Input: part model. Units: mm. Frame: model coordinates. A direction names the side the tool comes from. Coordinates: 2 decimals unless noted, no trailing zeros. Loops run counter-clockwise (first coordinate to the right, second up) from the corner with the lowest first, then second, coordinate; pieces in that order, holes last. Notation, with made-up numbers: (-6, -27.5) - (1, -27.5) arc R30 cw to (1, 10.5) - close; hole circle Ø11 at (-7.5, -29.5). An arc over 180 degrees is marked (long way). Use a Markdown table: item, result. Add a question column.
1. Section query C-C on z = -18. Return the cut outline in (x, y) (3 decimals), then the cut area to 3 significant figures.
2. Contact query for flat-ended pins moving along their axis: P1, Ø4, axis at x = 34.5, y = 0, coming from the -Z side (3 decimals); P2, Ø1.5, axis at y = 2, z = -17.5, coming from the +X side (3 decimals); P3, Ø4, axis at y = -2.5, z = -18.5, coming from the -X side (3 decimals). Output: stop coordinate, or through.
3. Access query for faces 4 (the face through (26, 0, -15.875)), 5 (the face through (45, 0, 15.875)), 6 (the face through (-27, 0, -15.875)). Directions: +Z, -Z, +X, -X, +Y, -Y. A direction counts if a zero-diameter tool reaches every point of the face in a straight line with its end or side. Return the directions, or none.
4. Section query A-A on z = 13.5. Return the cut outline in (x, y), then the cut area to 3 significant figures.
5. Section query B-B on y = 1.75. Return the cut outline in (x, z) (3 decimals), then the cut area to 3 significant figures.
6. Ray query, L1, parallel to X at y = -4, z = -16.5 (3 decimals); L2, parallel to Z at x = -42, y = -2 (3 decimals); L3, parallel to X at y = -2.75, z = 6.5. Return the intervals inside material, ascending. Write a range as [from, to].
7. Draft query along X for faces 1 (the face through (-0.63, -0.09, -3.17)), 2 (the face through (50.8, 0, 0)), 3 (the face through (-45, 0, 15.875)). Return one class per face: released by +X, released by -X, zero draft, split by the parting line, or undercut.
8. Section query D-D on x = 43.5. Return the cut outline in (y, z) (3 decimals), then the cut area to 3 significant figures.
```python
from build123d import *

# Parameters (mm, degrees)
F0_W     = 101.6
F0_H     = 31.75
F1_DEPTH = 6.35
F3_DEPTH = 12.7
F4_W     = 6.35
F4_H     = 12.7
F5_DEPTH = 6.35
F6_R     = 1.27


with BuildPart() as f1:
    # F0 (on Front) → F1 (new body, symmetric)
    with BuildSketch(Plane.XZ):
        Rectangle(F0_W, F0_H)
    extrude(amount=F1_DEPTH, both=True)

    # F2 (on Front) → F3 (cut, symmetric)
    with BuildSketch(Plane.XZ):
        with BuildLine():
            Line((39.6557372898, 15.875), (-39.6557372898, 15.875))
            ThreePointArc((-39.6557372898, 15.875), (0, -3.175), (39.6557372898, 15.875))
        make_face()
    extrude(amount=F3_DEPTH, both=True, mode=Mode.SUBTRACT)

    # F4 (on face) → F5 (join)
    with BuildSketch(Plane(origin=(0, 0, -15.875), x_dir=(1, 0, 0), z_dir=(0, 0, -1))):
        Rectangle(F4_W, F4_H)
    extrude(amount=F5_DEPTH)

    # F6
    f6_edges = [f1.edges().sort_by_distance(p)[0] for p in [
        (-3.175, 0, -22.225),
        (3.175, 0, -22.225),
        (-50.8, 0, -15.875),
        (-50.8, 0, 15.875),
        (-39.655737, 0, 15.875),
        (39.655737, 0, 15.875),
        (50.8, 0, 15.875),
        (50.8, 0, -15.875),
    ]]
    fillet(f6_edges, radius=F6_R)


solid = f1.part
```
Resolved:
| question | item | result |
|---|---|---|
| 1 | outline | (-3.175, -6.35) - (3.175, -6.35) - (3.175, 6.35) - (-3.175, 6.35) - close |
| 1 | area | 80.6 mm² |
| 2 | P1 | z = -15.875 |
| 2 | P2 | x = 3.175 |
| 2 | P3 | x = -3.175 |
| 3 | face 4 | -Z, +X, +Y, -Y |
| 3 | face 5 | +Z, +X, -X, +Y, -Y |
| 3 | face 6 | -Z, -X, +Y, -Y |
| 4 | outline | (-50.8, -6.35) - (-37.63, -6.35) - (-37.63, 6.35) - (-50.8, 6.35) - close; (37.63, -6.35) - (50.8, -6.35) - (50.8, 6.35) - (37.63, 6.35) - close |
| 4 | area | 334 mm² |
| 5 | outline | (-50.8, -14.605) arc R1.27 ccw to (-49.53, -15.875) - (-3.175, -15.875) - (-3.175, -20.955) arc R1.27 ccw to (-1.905, -22.225) - (1.905, -22.225) arc R1.27 ccw to (3.175, -20.955) - (3.175, -15.875) - (49.53, -15.875) arc R1.27 ccw to (50.8, -14.605) - (50.8, 14.605) arc R1.27 ccw to (49.53, 15.875) - (40.261, 15.875) arc R1.27 ccw to (39.279, 15.41) arc R50.8 cw to (-39.279, 15.41) arc R1.27 ccw to (-40.261, 15.875) - (-49.53, 15.875) arc R1.27 ccw to (-50.8, 14.605) - close |
| 5 | area | 2,210 mm² |
| 6 | L1 | [-3.175, 3.175] |
| 6 | L2 | [-15.875, 15.875] |
| 6 | L3 | [-50.8, -29.82], [29.82, 50.8] |
| 7 | face 1 | undercut |
| 7 | face 2 | released by +X |
| 7 | face 3 | zero draft |
| 8 | outline | (-6.35, -15.875) - (6.35, -15.875) - (6.35, 15.875) - (-6.35, 15.875) - close |
| 8 | area | 403 mm² |
